Verification items for the finished model (mm, model axes). A direction names the side the tool comes from. Coordinates: 2 decimals unless noted, no trailing zeros. Write each loop counter-clockwise with the first axis right and the second up, starting at its lowest first coordinate (ties: lowest second). Pieces come first, ordered by that corner, then holes. Notation, with made-up numbers: (-3.75, 49.5) -> (20.25, 49.5) arc R10 cw to (20.25, 66.5) -> close; hole circle Ø3 at (-4, 78.25). An arc over 180 degrees is marked (long way). Write each question's results on one line, items separated by ' | '. Start each with the question number.
from build123d import *


with BuildPart() as part:
    # Sketch1 → Revolve1 (revolve)
    with BuildSketch(Plane.XY, mode=Mode.PRIVATE) as revolve1_sk:
        with BuildLine():
            Line((0, 6.35), (-1.602370205, 6.35))
            Line((-1.602370205, 6.35), (-2.5, 3))
            Line((-2.5, 3), (-2.5, 1))
            ThreePointArc((-2.5, 1), (-1.5, 0), (-2.5, -1))
            Line((-2.5, -1), (-2.5, -6.35))
            Line((-2.5, -6.35), (-4.5, -6.35))
            Line((-4.5, -6.35), (-4.5, -7.35))
            Line((-4.5, -7.35), (0, -7.35))
            Line((0, -7.35), (0, 6.35))
        make_face()
    revolve(revolve1_sk.sketch.rotate(Axis((0, 0, 0), (0, 1, 0)), 270), axis=Axis((0, 0, 0), (0, 1, 0)))


solid = part.part
1. Sectioned sample at D-D on y = -5.75. Record the cut outline in (x, z).
2. Mould release check, pull along Y, two halves, no side actions. Record for faces 3 (the flat face through (2, -6.35, 2)), 4 (the cylindrical face through (2.44, 1.99, 0.54)), 5 (the flat face through (0, -7.35, 0)): +Y half, -Y half, draft (parallel to the pull), parting line (faces both ways), or undercut.
3. Sectioned sample at A-A on z = 0. Record the cut outline in (x, y), plus the area to 3 significant figures.
4. Tool access check on faces 1 (the flat face through (0, 6.35, 0)), 2 (the cylindrical face through (2.44, -3.71, 0.54)). Record the directions out of +Z, -Z, +X, -X, +Y, -Y that give a thin tool (end or side, any length) a straight path to the whole face; none if there is none.
5. Sectioned sample at B-B on x = 0. Record the cut outline in (y, z), plus the area to 3 significant figures.
6. Material ranges on probe 1 along Y at (x, z) = (4, -0.75); probe 2 along X at (y, z) = (4.5, 0.5); probe 3 along Z at (x, y) = (2, -4.5), recorded low to high. Write a range as from..to.
7. Depth check by flat-ended pin: pin 1 Ø4 at (x, y) = (1, 3.5) entering from +Z; pin 2 Ø1 at (x, y) = (1, 4.5) entering from -Z; pin 3 Ø1.5 at (y, z) = (4.5, 0) entering from -X. Enter the tip coordinate at first touch or a pass-through.
8. Sectioned sample at C-C on y = 0. Record the cut outline in (x, z).
Computed values:
1) outline: circle Ø5 at (0, 0)
2) face 3: +Y half | face 4: draft | face 5: -Y half
3) outline: (-4.5, -7.35) -> (4.5, -7.35) -> (4.5, -6.35) -> (2.5, -6.35) -> (2.5, -1) arc R1 cw to (2.5, 1) -> (2.5, 3) -> (1.6, 6.35) -> (-1.6, 6.35) -> (-2.5, 3) -> (-2.5, 1) arc R1 cw to (-2.5, -1) -> (-2.5, -6.35) -> (-4.5, -6.35) -> close | area: 66.4 mm^2
4) face 1: +Z, -Z, +X, -X, +Y | face 2: +Y
5) outline: (-7.35, -4.5) -> (-6.35, -4.5) -> (-6.35, -2.5) -> (-1, -2.5) arc R1 cw to (1, -2.5) -> (3, -2.5) -> (6.35, -1.6) -> (6.35, 1.6) -> (3, 2.5) -> (1, 2.5) arc R1 cw to (-1, 2.5) -> (-6.35, 2.5) -> (-6.35, 4.5) -> (-7.35, 4.5) -> close | area: 66.4 mm^2
6) probe 1: y = -7.35..-6.35 | probe 2: x = -2.04..2.04 | probe 3: z = -1.5..1.5
7) pin 1: stops at z = 2.5 | pin 2: stops at z = -2.1 | pin 3: stops at x = -2.3
8) outline: circle Ø3 at (0, 0)
